Build history of the part. All positions in model axes, mm. A direction names the side the tool comes from. Round coordinates to 2 decimals unless told otherwise and drop trailing zeros. Loops run counter-clockwise (first coordinate to the right, second up) from the corner with the lowest first, then second, coordinate; pieces in that order, holes last. Notation, with made-up numbers: M 78.5,8 L 136.5,8 A20 ccw 136.5,26 Z; hole C -19.5,-38 d1. An arc over 180 degrees is marked long. Write each question's results on one line, items separated by ' | '. Start each with the question number.
```python
from build123d import *

# Parameters (mm, degrees)
F0_W         = 127
F0_H         = 76.2
F1_DEPTH     = 25.4
F2_R         = 6.35
F3_DEPTH     = 25.401
F4_W         = 10.16
F4_H         = 25.4
F6_W         = 15.24
F6_H         = 12.7
F8_R         = 2.54
F9_R         = 1.27
F10_T1_DEPTH = 140.0641495789
F10_T3_DEPTH = 89.2641495789


# Not quite as in the source:
# - a fillet or chamfer that OpenCascade refuses, or shapes differently, is made with other operations: its cross-section is extruded or revolved along the edge and cut away or added


with BuildPart() as f1:
    # F0 (on Top) → F1 (new body)
    with BuildSketch(Plane.XY):
        Rectangle(F0_W, F0_H)
    extrude(amount=F1_DEPTH)

    # F2 (on face) → F3 (cut, through all)
    with BuildSketch(Plane.XY.offset(25.4)):
        with Locations((53.34, 27.94)):
            Circle(F2_R)
        with Locations((53.34, -27.94)):
            Circle(F2_R)
        with Locations((-53.34, 27.94)):
            Circle(F2_R)
        with Locations((-53.34, -27.94)):
            Circle(F2_R)
    extrude(amount=-F3_DEPTH, mode=Mode.SUBTRACT)

    # F4 (on Front) → F5 (revolve)
    with BuildSketch(Plane.XZ):
        with Locations((5.08, 38.1)):
            Rectangle(F4_W, F4_H)
    revolve(axis=Axis((0, 0, 38.1), (0, 0, -1)))

    # F6 (on Front) → F7 (revolve, cut)
    with BuildSketch(Plane.XZ):
        with Locations((12.7, 38.3218890125)):
            Rectangle(F6_W, F6_H)
    revolve(axis=Axis((0, 0, 25.4), (0, 0, 1)), mode=Mode.SUBTRACT)

    # F8
    f8_edges = [f1.edges().sort_by_distance(p)[0] for p in [
        (-10.16, 0, 50.8),
    ]]
    fillet(f8_edges, radius=F8_R)

    # F9
    f9_edges = [f1.edges().sort_by_distance(p)[0] for p in [
        (-10.16, 0, 31.971889),
        (-5.08, 0, 31.971889),
        (-10.16, 0, 25.4),
    ]]
    fillet(f9_edges, radius=F9_R)

    # F10: chamfer of 2.54 on 9 edges, made by hand

    # F10_s2 → F10_t1 (cut)
    with BuildSketch(Plane.YZ.offset(-70.0320747894)):
        Polygon((35.56, 25.4), (38.1, 22.86), (38.1, 25.4), align=None)
        Polygon((-35.56, 25.4), (-38.1, 22.86), (-38.1, 25.4), align=None)
    extrude(amount=F10_T1_DEPTH, mode=Mode.SUBTRACT)

    # F10_s4 → F10_t3 (cut)
    with BuildSketch(Plane.XZ.offset(-44.6320747894)):
        Polygon((60.96, 25.4), (63.5, 22.86), (63.5, 25.4), align=None)
        Polygon((-60.96, 25.4), (-63.5, 22.86), (-63.5, 25.4), align=None)
    extrude(amount=F10_T3_DEPTH, mode=Mode.SUBTRACT)

    # F10_s5 → F10_t6 (revolve, cut)
    with BuildSketch(Plane.XZ.offset(27.94)):
        Polygon((-44.45, 25.4), (-46.99, 22.86), (-46.99, 25.4), align=None)
    revolve(axis=Axis((-53.34, -27.94, 25.4), (0, 0, 1)), mode=Mode.SUBTRACT)

    # F10_s7 → F10_t8 (revolve, cut)
    with BuildSketch(Plane.XZ.offset(27.94)):
        Polygon((62.23, 25.4), (59.69, 22.86), (59.69, 25.4), align=None)
    revolve(axis=Axis((53.34, -27.94, 25.4), (0, 0, 1)), mode=Mode.SUBTRACT)

    # F10_s9 → F10_t10 (revolve, cut)
    with BuildSketch(Plane.XZ.offset(-27.94)):
        Polygon((-44.45, 25.4), (-46.99, 22.86), (-46.99, 25.4), align=None)
    revolve(axis=Axis((-53.34, 27.94, 25.4), (0, 0, 1)), mode=Mode.SUBTRACT)

    # F10_s11 → F10_t12 (revolve, cut)
    with BuildSketch(Plane.XZ.offset(-27.94)):
        Polygon((62.23, 25.4), (59.69, 22.86), (59.69, 25.4), align=None)
    revolve(axis=Axis((53.34, 27.94, 25.4), (0, 0, 1)), mode=Mode.SUBTRACT)


solid = f1.part
```
Item 1: Tool access for faces 5 (the flat face through (5, -2, 44.672)), 6 (the cylindrical face through (-1.323, -10.074, 46.491)), 7 (the cylindrical face through (-59.684, 28.219, 11.59)): list every direction of +Z, -Z, +X, -X, +Y, -Y with a clear straight run to the whole face (end or side of a thin tool).
Item 2: Mould opens along X. For faces 1 (the cylindrical face through (59.397, -26.033, 11.59)), 2 (the flat face through (62.21, 0.53, 24.15)), 3 (the flat face through (-62.21, 0.53, 24.15)), 4 (the cylindrical face through (-59.684, -27.661, 11.59)) say: released by +X, released by -X, zero draft, split by the parting line, or undercut.
Item 3: Saw through at D-D, the plane y = 0. Give the cut face in (x, z), then the cut area to 3 significant figures.
Item 4: Drill centre lines: line 1 along Y through (x, z) = (-53, 17); line 2 along X through (y, z) = (27, 24); line 3 along X through (y, z) = (27, 5). Where is each one in solid material? Low to high. Write a range as [from, to].
Item 5: Saw through at A-A, the plane z = 15. Give the cut face in (x, y), then the cut area to 3 significant figures.
Item 6: Drop flat-ended pins along their axis: pin 1 (3.5 mm diameter, centred on x = -59, y = -33.5, fed in from +Z); pin 2 (10 mm diameter, centred on x = 4, y = 3.5, fed in from -Z); pin 3 (1.5 mm diameter, centred on x = 58.5, y = 33.5, fed in from +Z); pin 4 (14.5 mm diameter, centred on x = 53.34, y = -27.94, fed in from +Z). Give the stop position or say it passes through.
Item 7: Saw through at B-B, the plane y = 27.94. Give the cut face in (x, z) (3 decimals).
Item 8: Saw through at C-C, the plane x = -53.34. Give the cut face in (y, z) (3 decimals).
Working result:
1) face 5: none | face 6: +Z | face 7: +Z, -Z
2) face 1: undercut | face 2: released by +X | face 3: released by -X | face 4: undercut
3) outline: M -63.5,0 L 63.5,0 L 63.5,22.86 L 60.96,25.4 L 11.43,25.4 A1.27 cw 10.16,26.67 L 10.16,30.7 A1.27 ccw 8.89,31.97 L 6.35,31.97 A1.27 cw 5.08,33.24 L 5.08,44.67 L 10.16,44.67 L 10.16,48.26 A2.54 ccw 7.62,50.8 L -7.62,50.8 A2.54 ccw -10.16,48.26 L -10.16,44.67 L -5.08,44.67 L -5.08,33.24 A1.27 cw -6.35,31.97 L -8.89,31.97 A1.27 ccw -10.16,30.7 L -10.16,26.67 A1.27 cw -11.43,25.4 L -60.96,25.4 L -63.5,22.86 Z | area: 3,600 mm²
4) line 1: y = [-38.1, -34.28], [-21.6, 21.6], [34.28, 38.1] | line 2: x = [-62.36, -60.77], [-45.91, 45.91], [60.77, 62.36] | line 3: x = [-63.5, -59.62], [-47.06, 47.06], [59.62, 63.5]
5) outline: M -63.5,-38.1 L 63.5,-38.1 L 63.5,38.1 L -63.5,38.1 Z; hole C -53.34,-27.94 d12.7; hole C -53.34,27.94 d12.7; hole C 53.34,-27.94 d12.7; hole C 53.34,27.94 d12.7 | area: 9,170 mm²
6) pin 1: stops at z = 25.4 | pin 2: stops at z = 0 | pin 3: stops at z = 24.85 | pin 4: stops at z = 23.76
7) outline: M -63.5,0 L -59.69,0 L -59.69,22.86 L -61.595,24.765 L -63.5,22.86 Z; M -46.99,0 L 46.99,0 L 46.99,22.86 L 44.45,25.4 L -44.45,25.4 L -46.99,22.86 Z; M 59.69,0 L 63.5,0 L 63.5,22.86 L 61.595,24.765 L 59.69,22.86 Z
8) outline: M -38.1,0 L -34.29,0 L -34.29,22.86 L -36.195,24.765 L -38.1,22.86 Z; M -21.59,0 L 21.59,0 L 21.59,22.86 L 19.05,25.4 L -19.05,25.4 L -21.59,22.86 Z; M 34.29,0 L 38.1,0 L 38.1,22.86 L 36.195,24.765 L 34.29,22.86 Z
